Geometry: final body of the model. Coordinates: model frame, mm. A direction names the side the tool comes from. Give positions to 0.01 mm unless a question says otherwise; leave off trailing zeros. Write each loop counter-clockwise with the first axis right and the second up, starting at its lowest first coordinate (ties: lowest second). Pieces come first, ordered by that corner, then holes. Notation, with made-up numbers: (56, 65) - (113, 65) arc R18 ccw to (113, 79) - close; hole circle Ø9 at (58.5, 60.25). An arc over 180 degrees is marked (long way). Return JSON: item names as keys, results as strings.
from build123d import *

# Parameters (mm, degrees)
F0_R     = 2.5
F1_DEPTH = 20
F2_DEPTH = 1
F3_R     = 35
F3_R_2   = 1.5
F3_R_3   = 2.5
F4_DEPTH = 1
F5_DEPTH = 7
F8_DEPTH = 3


with BuildPart() as f1:
    # F0 (on Front) → F1 (new body)
    with BuildSketch(Plane.XZ):
        with BuildLine():
            ThreePointArc((5.5655123118, 2.2416673945), (20.6488442828, 5.9277985889), (35, 0))
            ThreePointArc((35, 0), (20.2866870884, 9.5155994681), (3.3649940235, 4.9675763931))
            ThreePointArc((3.3649940235, 4.9675763931), (2.8709960308, 5.2685274784), (2.3503132806, 5.5205097122))
            ThreePointArc((2.3503132806, 5.5205097122), (10.4093512363, 18.7925243957), (24.7487373415, 24.7487373415))
            ThreePointArc((24.7487373415, 24.7487373415), (7.6163090971, 21.073398919), (-1.133196861, 5.8920170463))
            ThreePointArc((-1.133196861, 5.8920170463), (-1.6953107447, 5.755512269), (-2.2416673945, 5.5655123118))
            ThreePointArc((-2.2416673945, 5.5655123118), (-5.9277985889, 20.6488442828), (0, 35))
            ThreePointArc((0, 35), (-9.5155994681, 20.2866870884), (-4.9675763931, 3.3649940235))
            ThreePointArc((-4.9675763931, 3.3649940235), (-5.2685274784, 2.8709960308), (-5.5205097122, 2.3503132806))
            ThreePointArc((-5.5205097122, 2.3503132806), (-18.7925243957, 10.4093512363), (-24.7487373415, 24.7487373415))
            ThreePointArc((-24.7487373415, 24.7487373415), (-21.073398919, 7.6163090971), (-5.8920170463, -1.133196861))
            ThreePointArc((-5.8920170463, -1.133196861), (-5.755512269, -1.6953107447), (-5.5655123118, -2.2416673945))
            ThreePointArc((-5.5655123118, -2.2416673945), (-20.6488442828, -5.9277985889), (-35, 0))
            ThreePointArc((-35, 0), (-20.2866870884, -9.5155994681), (-3.3649940235, -4.9675763931))
            ThreePointArc((-3.3649940235, -4.9675763931), (-2.8709960308, -5.2685274784), (-2.3503132806, -5.5205097122))
            ThreePointArc((-2.3503132806, -5.5205097122), (-10.4093512363, -18.7925243957), (-24.7487373415, -24.7487373415))
            ThreePointArc((-24.7487373415, -24.7487373415), (-7.6163090971, -21.073398919), (1.133196861, -5.8920170463))
            ThreePointArc((1.133196861, -5.8920170463), (1.6953107447, -5.755512269), (2.2416673945, -5.5655123118))
            ThreePointArc((2.2416673945, -5.5655123118), (5.9277985889, -20.6488442828), (0, -35))
            ThreePointArc((0, -35), (9.5155994681, -20.2866870884), (4.9675763931, -3.3649940235))
            ThreePointArc((4.9675763931, -3.3649940235), (5.2685274784, -2.8709960308), (5.5205097122, -2.3503132806))
            ThreePointArc((5.5205097122, -2.3503132806), (18.7925243957, -10.4093512363), (24.7487373415, -24.7487373415))
            ThreePointArc((24.7487373415, -24.7487373415), (21.073398919, -7.6163090971), (5.8920170463, 1.133196861))
            ThreePointArc((5.8920170463, 1.133196861), (5.755512269, 1.6953107447), (5.5655123118, 2.2416673945))
        make_face()
        Circle(F0_R, mode=Mode.SUBTRACT)
    extrude(amount=F1_DEPTH)

    # F0 (on Front) → F2 (join)
    with BuildSketch(Plane.XZ):
        with BuildLine():
            ThreePointArc((3.3649940235, 4.9675763931), (20.2866870884, 9.5155994681), (35, 0))
            ThreePointArc((35, 0), (32.3357836379, 13.3939201328), (24.7487373415, 24.7487373415))
            ThreePointArc((24.7487373415, 24.7487373415), (10.4093512363, 18.7925243957), (2.3503132806, 5.5205097122))
            ThreePointArc((2.3503132806, 5.5205097122), (2.8709960308, 5.2685274784), (3.3649940235, 4.9675763931))
        make_face()
        with BuildLine():
            ThreePointArc((5.5655123118, 2.2416673945), (20.6488442828, 5.9277985889), (35, 0))
            ThreePointArc((35, 0), (20.2866870884, 9.5155994681), (3.3649940235, 4.9675763931))
            ThreePointArc((3.3649940235, 4.9675763931), (2.8709960308, 5.2685274784), (2.3503132806, 5.5205097122))
            ThreePointArc((2.3503132806, 5.5205097122), (10.4093512363, 18.7925243957), (24.7487373415, 24.7487373415))
            ThreePointArc((24.7487373415, 24.7487373415), (7.6163090971, 21.073398919), (-1.133196861, 5.8920170463))
            ThreePointArc((-1.133196861, 5.8920170463), (-1.6953107447, 5.755512269), (-2.2416673945, 5.5655123118))
            ThreePointArc((-2.2416673945, 5.5655123118), (-5.9277985889, 20.6488442828), (0, 35))
            ThreePointArc((0, 35), (-9.5155994681, 20.2866870884), (-4.9675763931, 3.3649940235))
            ThreePointArc((-4.9675763931, 3.3649940235), (-5.2685274784, 2.8709960308), (-5.5205097122, 2.3503132806))
            ThreePointArc((-5.5205097122, 2.3503132806), (-18.7925243957, 10.4093512363), (-24.7487373415, 24.7487373415))
            ThreePointArc((-24.7487373415, 24.7487373415), (-21.073398919, 7.6163090971), (-5.8920170463, -1.133196861))
            ThreePointArc((-5.8920170463, -1.133196861), (-5.755512269, -1.6953107447), (-5.5655123118, -2.2416673945))
            ThreePointArc((-5.5655123118, -2.2416673945), (-20.6488442828, -5.9277985889), (-35, 0))
            ThreePointArc((-35, 0), (-20.2866870884, -9.5155994681), (-3.3649940235, -4.9675763931))
            ThreePointArc((-3.3649940235, -4.9675763931), (-2.8709960308, -5.2685274784), (-2.3503132806, -5.5205097122))
            ThreePointArc((-2.3503132806, -5.5205097122), (-10.4093512363, -18.7925243957), (-24.7487373415, -24.7487373415))
            ThreePointArc((-24.7487373415, -24.7487373415), (-7.6163090971, -21.073398919), (1.133196861, -5.8920170463))
            ThreePointArc((1.133196861, -5.8920170463), (1.6953107447, -5.755512269), (2.2416673945, -5.5655123118))
            ThreePointArc((2.2416673945, -5.5655123118), (5.9277985889, -20.6488442828), (0, -35))
            ThreePointArc((0, -35), (9.5155994681, -20.2866870884), (4.9675763931, -3.3649940235))
            ThreePointArc((4.9675763931, -3.3649940235), (5.2685274784, -2.8709960308), (5.5205097122, -2.3503132806))
            ThreePointArc((5.5205097122, -2.3503132806), (18.7925243957, -10.4093512363), (24.7487373415, -24.7487373415))
            ThreePointArc((24.7487373415, -24.7487373415), (21.073398919, -7.6163090971), (5.8920170463, 1.133196861))
            ThreePointArc((5.8920170463, 1.133196861), (5.755512269, 1.6953107447), (5.5655123118, 2.2416673945))
        make_face()
        Circle(F0_R, mode=Mode.SUBTRACT)
        with BuildLine():
            ThreePointArc((24.7487373415, -24.7487373415), (32.3357836379, -13.3939201328), (35, 0))
            ThreePointArc((35, 0), (20.6488442828, 5.9277985889), (5.5655123118, 2.2416673945))
            ThreePointArc((5.5655123118, 2.2416673945), (5.755512269, 1.6953107447), (5.8920170463, 1.133196861))
            ThreePointArc((5.8920170463, 1.133196861), (21.073398919, -7.6163090971), (24.7487373415, -24.7487373415))
        make_face()
        with BuildLine():
            ThreePointArc((-1.133196861, 5.8920170463), (7.6163090971, 21.073398919), (24.7487373415, 24.7487373415))
            ThreePointArc((24.7487373415, 24.7487373415), (13.3939201328, 32.3357836379), (0, 35))
            ThreePointArc((0, 35), (-5.9277985889, 20.6488442828), (-2.2416673945, 5.5655123118))
            ThreePointArc((-2.2416673945, 5.5655123118), (-1.6953107447, 5.755512269), (-1.133196861, 5.8920170463))
        make_face()
        with BuildLine():
            ThreePointArc((0, -35), (13.3939201328, -32.3357836379), (24.7487373415, -24.7487373415))
            ThreePointArc((24.7487373415, -24.7487373415), (18.7925243957, -10.4093512363), (5.5205097122, -2.3503132806))
            ThreePointArc((5.5205097122, -2.3503132806), (5.2685274784, -2.8709960308), (4.9675763931, -3.3649940235))
            ThreePointArc((4.9675763931, -3.3649940235), (9.5155994681, -20.2866870884), (0, -35))
        make_face()
        with BuildLine():
            ThreePointArc((-4.9675763931, 3.3649940235), (-9.5155994681, 20.2866870884), (0, 35))
            ThreePointArc((0, 35), (-13.3939201328, 32.3357836379), (-24.7487373415, 24.7487373415))
            ThreePointArc((-24.7487373415, 24.7487373415), (-18.7925243957, 10.4093512363), (-5.5205097122, 2.3503132806))
            ThreePointArc((-5.5205097122, 2.3503132806), (-5.2685274784, 2.8709960308), (-4.9675763931, 3.3649940235))
        make_face()
        with BuildLine():
            ThreePointArc((-24.7487373415, -24.7487373415), (-13.3939201328, -32.3357836379), (0, -35))
            ThreePointArc((0, -35), (5.9277985889, -20.6488442828), (2.2416673945, -5.5655123118))
            ThreePointArc((2.2416673945, -5.5655123118), (1.6953107447, -5.755512269), (1.133196861, -5.8920170463))
            ThreePointArc((1.133196861, -5.8920170463), (-7.6163090971, -21.073398919), (-24.7487373415, -24.7487373415))
        make_face()
        with BuildLine():
            ThreePointArc((-5.8920170463, -1.133196861), (-21.073398919, 7.6163090971), (-24.7487373415, 24.7487373415))
            ThreePointArc((-24.7487373415, 24.7487373415), (-32.3357836379, 13.3939201328), (-35, 0))
            ThreePointArc((-35, 0), (-20.6488442828, -5.9277985889), (-5.5655123118, -2.2416673945))
            ThreePointArc((-5.5655123118, -2.2416673945), (-5.755512269, -1.6953107447), (-5.8920170463, -1.133196861))
        make_face()
        with BuildLine():
            ThreePointArc((-35, 0), (-32.3357836379, -13.3939201328), (-24.7487373415, -24.7487373415))
            ThreePointArc((-24.7487373415, -24.7487373415), (-10.4093512363, -18.7925243957), (-2.3503132806, -5.5205097122))
            ThreePointArc((-2.3503132806, -5.5205097122), (-2.8709960308, -5.2685274784), (-3.3649940235, -4.9675763931))
            ThreePointArc((-3.3649940235, -4.9675763931), (-20.2866870884, -9.5155994681), (-35, 0))
        make_face()
    extrude(amount=-F2_DEPTH)

    # F3 (on face) → F4 (join)
    with BuildSketch(Plane.XZ.offset(20)):
        Circle(F3_R)
        with Locations((-4.5, 0)):
            Circle(F3_R_2, mode=Mode.SUBTRACT)
        Circle(F3_R_3, mode=Mode.SUBTRACT)
        with Locations((4.5, 0)):
            Circle(F3_R_2, mode=Mode.SUBTRACT)
    extrude(amount=F4_DEPTH)

    # F5 (add): faces of the model
    f5_faces = [f1.faces().sort_by_distance(p)[0] for p in [
        (4.5, -20, 0),
        (-4.5, -20, 0),
    ]]
    extrude(f5_faces, amount=F5_DEPTH)

    # F6 (on face) + F7 (on face) → F8 (cut)
    with BuildSketch(Plane.XZ.offset(27)):
        with BuildLine():
            Line((-3.0857864376, 0.5), (-5.9142135624, 0.5))
            ThreePointArc((-5.9142135624, 0.5), (-5.9783978395, 0.2536529681), (-6, 0))
            ThreePointArc((-6, 0), (-5.9783978395, -0.2536529681), (-5.9142135624, -0.5))
            Line((-5.9142135624, -0.5), (-3.0857864376, -0.5))
            ThreePointArc((-3.0857864376, -0.5), (-3.0216021605, -0.2536529681), (-3, 0))
            ThreePointArc((-3, 0), (-3.0216021605, 0.2536529681), (-3.0857864376, 0.5))
        make_face()
        with BuildLine():
            Line((-3, 0.5), (-3.0857864376, 0.5))
            ThreePointArc((-3.0857864376, 0.5), (-3.0216021605, 0.2536529681), (-3, 0))
            Line((-3, 0), (-3, 0.5))
        make_face()
    with BuildSketch(Plane.XZ.offset(27)):
        with BuildLine():
            Line((5.9142135624, 0.5), (3.0857864376, 0.5))
            ThreePointArc((3.0857864376, 0.5), (3.0216021605, 0.2536529681), (3, 0))
            ThreePointArc((3, 0), (3.0216021605, -0.2536529681), (3.0857864376, -0.5))
            Line((3.0857864376, -0.5), (5.9142135624, -0.5))
            ThreePointArc((5.9142135624, -0.5), (5.9783978395, -0.2536529681), (6, 0))
            ThreePointArc((6, 0), (5.9783978395, 0.2536529681), (5.9142135624, 0.5))
        make_face()
        with BuildLine():
            Line((6, 0.5), (5.9142135624, 0.5))
            ThreePointArc((5.9142135624, 0.5), (5.9783978395, 0.2536529681), (6, 0))
            Line((6, 0), (6, 0.5))
        make_face()
    extrude(amount=-F8_DEPTH, mode=Mode.SUBTRACT)


solid = f1.part
Q1. Mould query, pull axis X, two halves, no side actions, for faces 1 (the cylindrical face through (-0.54, -9.85, -2.44)), 2 (the flat face through (5, -26, 0.5)). Classes: pulls with the +X half, pulls with the -X half, needs draft (parallel to the pull), parting line crosses it, or undercut.
Answer key:
{"face 1": "undercut", "face 2": "needs draft"}
Q2. Pin query (flat end, axial travel): P1, Ø2, axis at x = -22, z = -10, coming from the -Y side; P2, Ø1, axis at y = -5, z = 22, coming from the +X side; P3, Ø0.8, axis at x = -5, z = 0, coming from the -Y side. Return the tip coordinate at first contact, or that it passes through.
Answer key:
{"P1": "stops at y = -21", "P2": "stops at x = 16.17", "P3": "stops at y = -24"}
Q3. Section query B-B, the plane z = -22. Return the cut outline in (x, y).
Answer key:
{"outline": "(-27.22, -21) - (27.22, -21) - (27.22, -20) - (25.14, -20) - (25.14, 0) - (27.22, 0) - (27.22, 1) - (-27.22, 1) - (-27.22, 0) - (-15.15, 0) - (-15.15, -20) - (-27.22, -20) - close; hole (-9, -20) - (5.79, -20) - (5.79, 0) - (-9, 0) - close; hole (9.17, -20) - (24.38, -20) - (24.38, 0) - (9.17, 0) - close"}
Q4. Section query C-C, the plane x = -22. Return the cut outline in (y, z).
Answer key:
{"outline": "(-21, -27.22) - (-20, -27.22) - (-20, -25.14) - (0, -25.14) - (0, -27.22) - (1, -27.22) - (1, 27.22) - (0, 27.22) - (0, 15.15) - (-20, 15.15) - (-20, 27.22) - (-21, 27.22) - close; hole (-20, -24.38) - (0, -24.38) - (0, -9.17) - (-20, -9.17) - close; hole (-20, -5.79) - (0, -5.79) - (0, 9) - (-20, 9) - close"}
Q5. Material intervals for probe 1 along Y at (x, z) = (17, -12); probe 2 along Z at (x, y) = (-4, -9.75); probe 3 along Z at (x, y) = (21, -15.5), sorted ascending. Write a range as [from, to].
Answer key:
{"probe 1": "y = [-21, -20], [0, 1]", "probe 2": "z = [-17.75, -10.31], [-5.46, 8.95], [28.55, 31.63]", "probe 3": "z = [-13.41, -7.52], [5.9, 9.39], [24.17, 25.2]"}
Q6. Section query D-D, the plane x = 30. Return the cut outline in (y, z).
Answer key:
{"outline": "(-21, -18.03) - (-20, -18.03) - (-20, 3.33) - (0, 3.33) - (0, -18.03) - (1, -18.03) - (1, 18.03) - (0, 18.03) - (0, 5.37) - (-20, 5.37) - (-20, 18.03) - (-21, 18.03) - close"}
Q7. Set-up query: faces 3 (the cylindrical face through (-3.81, -23.96, -1.33)), 4 (the flat face through (-4, -26, 0.5)), 5 (the cylindrical face through (20.428, -9.86, 5.944)). Return all of +Z, -Z, +X, -X, +Y, -Y with unobstructed straight access to the full face (end or side cutting, diameter ignored); none if empty.
Answer key:
{"face 3": "-Y", "face 4": "+X, -X, -Y", "face 5": "none"}
